Work out the finished part from the listing and answer in its coordinate system (mm). A direction names the side the tool comes from. Round coordinates to 2 decimals unless told otherwise and drop trailing zeros.
from build123d import *

# Parameters (mm, degrees)
SKETCH_1_W          = 150
SKETCH_1_H          = 5
EXTRUDE_1_DEPTH     = 1.5
SKETCH_2_W          = 12
SKETCH_2_H          = 3
EXTRUDE_2_DEPTH     = 3
SKETCH_3_R          = 1
CUT_EXTRUDE_1_DEPTH = 76.261211789
SKETCH_4_R          = 1.1
CUT_EXTRUDE_2_DEPTH = 76.261211789


with BuildPart() as part:
    # 草图1 → 凸台-拉伸1 (new, symmetric)
    with BuildSketch(Plane(origin=(0, 0, 0), x_dir=(1, 0, 0), z_dir=(0, 1, 0))):
        Rectangle(SKETCH_1_W, SKETCH_1_H)
    extrude(amount=EXTRUDE_1_DEPTH, both=True)

    # 草图2 → 凸台-拉伸2 (add)
    with BuildSketch(Plane(origin=(0, 1.5, 0), x_dir=(1, 0, 0), z_dir=(0, 1, 0))):
        with Locations((-60, -4)):
            Rectangle(SKETCH_2_W, SKETCH_2_H)
        with Locations((-30, -4)):
            Rectangle(SKETCH_2_W, SKETCH_2_H)
        with Locations((0, -4)):
            Rectangle(SKETCH_2_W, SKETCH_2_H)
        with Locations((30, -4)):
            Rectangle(SKETCH_2_W, SKETCH_2_H)
        with Locations((60, -4)):
            Rectangle(SKETCH_2_W, SKETCH_2_H)
    extrude(amount=-EXTRUDE_2_DEPTH)

    # 草图3 → 切除-拉伸1 (cut, through all)
    with BuildSketch(Plane.XZ.offset(1.5)):
        with Locations((67, 2.5)):
            Circle(SKETCH_3_R)
        with Locations((53, 2.5)):
            Circle(SKETCH_3_R)
        with Locations((37, 2.5)):
            Circle(SKETCH_3_R)
        with Locations((23, 2.5)):
            Circle(SKETCH_3_R)
        with Locations((7, 2.5)):
            Circle(SKETCH_3_R)
        with Locations((-7, 2.5)):
            Circle(SKETCH_3_R)
        with Locations((-23, 2.5)):
            Circle(SKETCH_3_R)
        with Locations((-37, 2.5)):
            Circle(SKETCH_3_R)
        with Locations((-53, 2.5)):
            Circle(SKETCH_3_R)
        with Locations((-67, 2.5)):
            Circle(SKETCH_3_R)
    extrude(amount=-CUT_EXTRUDE_1_DEPTH, mode=Mode.SUBTRACT)

    # 草图4 → 切除-拉伸2 (cut, through all)
    with BuildSketch(Plane(origin=(0, 1.5, 0), x_dir=(1, 0, 0), z_dir=(0, 1, 0))):
        with Locations(Location((63, -0.5, 0), (0, 0, 270))):
            Circle(SKETCH_4_R)
        with Locations(Location((57, -0.5, 0), (0, 0, 90))):
            Circle(SKETCH_4_R)
        with Locations(Location((-57, -0.5, 0), (0, 0, 270))):
            Circle(SKETCH_4_R)
        with Locations(Location((-63, -0.5, 0), (0, 0, 90))):
            Circle(SKETCH_4_R)
    extrude(amount=-CUT_EXTRUDE_2_DEPTH, mode=Mode.SUBTRACT)


solid = part.part
Item 1: Find the intervals of material crossed by line 1 along X through (y, z) = (0.35, 5); line 2 along X through (y, z) = (0.4, 0.25); line 3 along Z through (x, y) = (57, -0.7), in increasing order.
Item 2: For a pull along X with two mould halves and no side action, classify faces 4 (the face through (-45, 0, 2.5)), 5 (the face through (-54, 0, 4)), 6 (the face through (-60, 0, 5.5)), 7 (the face through (-75, 0, 0)) as released by +X, released by -X, zero draft, split by the parting line, or undercut.
Item 3: Given pin 1 (0.9 mm diameter, centred on y = 0.5, z = 3.5, fed in from -X); pin 2 (1.5 mm diameter, centred on y = 0.5, z = 4.5, fed in from +X); pin 3 (1 mm diameter, centred on x = -9.5, y = 1, fed in from +Z), each flat-ended and moving along its own axis, determine where each tip first touches the part or whether it passes through.
Item 4: Find section A-A (y = 1.05). State how many separate pieces and enclosed holes the cut face has, plus the area to 3 significant figures.
Item 5: A tool of negligible diameter and unlimited length cuts with its end or side. For faces 1 (the face through (24, 0, 4)), 2 (the face through (-66, 0, 4)), 3 (the face through (66, 0, 4)), from which of +Z, -Z, +X, -X, +Y, -Y can it reach the whole face along a straight path? Write none if from no direction.
Model answer:
1. line 1: x = -66 to -54, -36 to -24, -6 to 6, 24 to 36, 54 to 66
1. line 2: x = -75 to -64.07, -61.93 to -58.07, -55.93 to 55.93, 58.07 to 61.93, 64.07 to 75
1. line 3: z = -2.5 to -0.6, 1.6 to 5.5
2. face 4: undercut
2. face 5: undercut
2. face 6: zero draft
2. face 7: released by -X
3. pin 1: stops at x = -66
3. pin 2: stops at x = 66
3. pin 3: stops at z = 2.5
4. separate pieces: 1
4. enclosed holes: 4
4. area: 899 mm2
5. face 1: +Z, +Y, -Y
5. face 2: +Z, -X, +Y, -Y
5. face 3: +Z, +X, +Y, -Y
